Work out the finished part from the listing and answer in its coordinate system (mm). Coordinates: 2 decimals unless noted, no trailing zeros. Order: outer loops, then holes, each group sorted by start corner. A loop starts at its lowest first (then second) coordinate and runs counter-clockwise, first axis right, second up. Notation, with made-up numbers: (85, -28.75) - (103, -28.75) arc R10 ccw to (103, -23.75) - close; hole circle Ø8 at (-7.5, 21). An arc over 180 degrees is marked (long way). Answer as a JSON object with one key per item and string values. Group by question number.
1) This flat-tipped pin is pushed along its axis until it touches: P1, Ø1.5, axis at x = 9, y = 2.5, coming from the +Z side. Where does it stop, or does it pass through?
2) Section C-C (x = -11) is taken. Give the vertices of the cut face in (y, z), plus the area to 3 significant figures.
3) Section A-A (z = 14.25) is taken. Give the vertices of the cut face in (x, y).
4) Section B-B (y = 2) is taken. Give the vertices of the cut face in (x, z), plus the area to 3 significant figures.
5) Find the intervals of material crossed by line 1 along X through (y, z) = (1.3, 11); line 2 along X through (y, z) = (2.9, 19.75); line 3 along Z through (x, y) = (-15.5, 1.35), in increasing order.
from build123d import *

# Parameters (mm, degrees)
RESSALTO_EXTRUS_O1_DEPTH = 3
ESBO_O2_W                = 30
ESBO_O2_H                = 16.142769795
CORTE_EXTRUS_O2_DEPTH    = 3


with BuildPart() as part:
    # Esboço1 → Ressalto-extrusão1 (new body)
    with BuildSketch(Plane(origin=(0, 0, 0), x_dir=(1, 0, 0), z_dir=(0, 1, 0))):
        Polygon((36, 7.331730769), (-39, 7.331730769), (-39, -22.668269231), (-3, -22.668269231), (-3, -7.668269231), (0, -7.668269231), (0, -22.668269231), (36, -22.668269231), align=None)
    extrude(amount=RESSALTO_EXTRUS_O1_DEPTH)

    # Esboço2 → Corte-extrusão2 (cut)
    with BuildSketch(Plane.XY.offset(22.668269231)):
        with Locations((-1.5, 0.209360247)):
            Rectangle(ESBO_O2_W, ESBO_O2_H)
    extrude(amount=-CORTE_EXTRUS_O2_DEPTH, mode=Mode.SUBTRACT)


solid = part.part
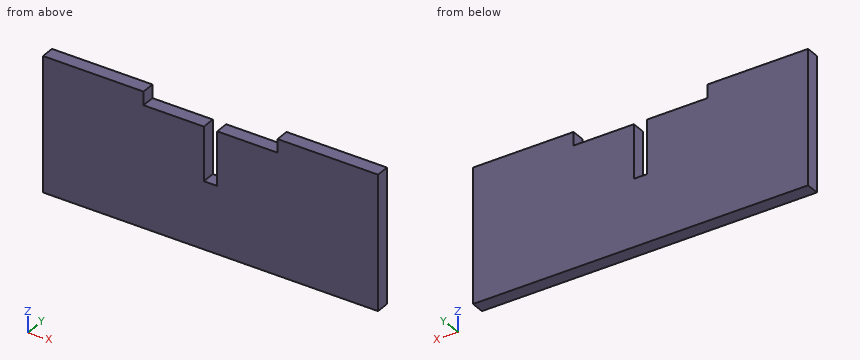
Report:
{
 "1": {"P1": "stops at z = 19.67"},
 "2": {"outline": "(0, -7.33) - (3, -7.33) - (3, 19.67) - (0, 19.67) - close", "area": "81.0 mm²"},
 "3": {"outline": "(-39, 0) - (-3, 0) - (-3, 3) - (-39, 3) - close; (0, 0) - (36, 0) - (36, 3) - (0, 3) - close"},
 "4": {"outline": "(-39, -7.33) - (36, -7.33) - (36, 22.67) - (13.5, 22.67) - (13.5, 19.67) - (0, 19.67) - (0, 7.67) - (-3, 7.67) - (-3, 19.67) - (-16.5, 19.67) - (-16.5, 22.67) - (-39, 22.67) - close", "area": "2,120 mm²"},
 "5": {"line 1": "x = -39 to -3, 0 to 36", "line 2": "x = -39 to -16.5, 13.5 to 36", "line 3": "z = -7.33 to 19.67"}
}
